Here's the drawing with two shaded views (mm, measured from the low corner). I have some questions. A direction names the side the tool comes from. Give positions to 0.01 mm unless a question says otherwise; leave off trailing zeros. Loops run counter-clockwise (first coordinate to the right, second up) from the corner with the lowest first, then second, coordinate; pieces in that order, holes last. Notation, with made-up numbers: M 85.25,27 L 142.25,27 A15 cw 142.25,42 Z; hole C -18.75,6 d8. An arc over 180 degrees is marked long. Use CSV: the item, a comma, the result in double quotes.
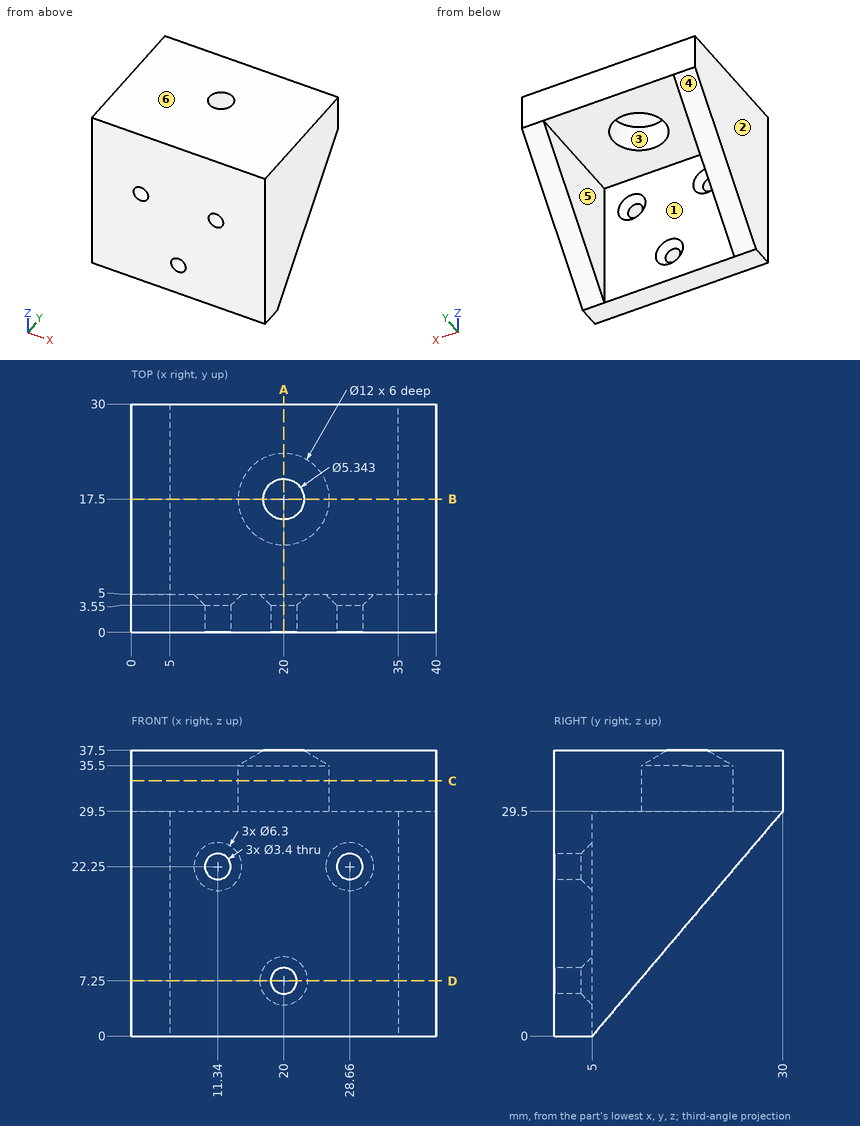
1. I want a section at B-B, the plane y = 17.5. List the corners of the cut face in (x, z) for me, then the cut area to 3 significant figures.
Outcome:
outline,"M 0,14.75 L 5,14.75 L 5,29.5 L 14,29.5 L 14,35.5 L 17.33,37.5 L 0,37.5 Z; M 22.67,37.5 L 26,35.5 L 26,29.5 L 35,29.5 L 35,14.75 L 40,14.75 L 40,37.5 Z"
area,"378 mm2"
2. I want a section at C-C, the plane z = 33.5. List the corners of the cut face in (x, y) for me, then the cut area to 3 significant figures.
Outcome:
outline,"M 0,0 L 40,0 L 40,30 L 0,30 Z; hole C 20,17.5 d12"
area,"1,090 mm2"
3. I'm going to push flat-ended pins straight in: pin 1 Ø5.5 at (x, z) = (20, 7.25) entering from +Y; pin 2 Ø4 at (x, z) = (32, 14) entering from +Y; pin 3 Ø8 at (x, y) = (6, 10.5) entering from -Z. Where does each tip first touch, or does it pass through?
Outcome:
pin 1,"y = 4.6"
pin 2,"y = 5"
pin 3,"z = 1.92"
4. If we mould it in two halves opening along X, with no side actions, what happens to the marked faces 1, 2, 3 and 4? For each: +X half, -X half, draft (parallel to the pull), parting line (faces both ways), or undercut.
Outcome:
face 1,"undercut"
face 2,"-X half"
face 3,"undercut"
face 4,"draft"
5. Which directions (+Z, -Z, +X, -X, +Y, -Y) give clear straight access to the entire face, cutting with the end or side of a thin tool? Please do the marked faces 5 and 6.
Outcome:
face 5,"-Z, +Y"
face 6,"+Z, +X, -X, +Y, -Y"
6. I want a section at D-D, the plane z = 7.25. List the corners of the cut face in (x, y) for me, then the cut area to 3 significant figures.
Outcome:
outline,"M 0,0 L 18.3,0 L 18.3,3.55 L 16.85,5 L 5,5 L 5,11.14 L 0,11.14 Z; M 21.7,0 L 40,0 L 40,11.14 L 35,11.14 L 35,5 L 23.15,5 L 21.7,3.55 Z"
area,"242 mm2"
7. Please list where these lines run through material, in increasing order: line 1 (X direction, y = 22, z = 22.5); line 2 (X direction, y = 1.5, z = 23) (1 decimal); line 3 (Z direction, x = 13, y = 6).
Outcome:
line 1,"0 to 5, 35 to 40"
line 2,"0 to 9.8, 12.9 to 27.1, 30.2 to 40"
line 3,"29.5 to 37.5"
8. I want a section at A-A, the plane x = 20. List the corners of the cut face in (y, z) for me, then the cut area to 3 significant figures.
Outcome:
outline,"M 0,0 L 5,0 L 5,4.1 L 3.55,5.55 L 0,5.55 Z; M 0,8.95 L 3.55,8.95 L 5,10.4 L 5,29.5 L 11.5,29.5 L 11.5,35.5 L 14.83,37.5 L 0,37.5 Z; M 20.17,37.5 L 23.5,35.5 L 23.5,29.5 L 30,29.5 L 30,37.5 Z"
area,"279 mm2"
